Model file for the job. Use its own axes, mm. A direction names the side the tool comes from. Round coordinates to 2 decimals unless told otherwise and drop trailing zeros. Write each loop counter-clockwise with the first axis right and the second up, starting at its lowest first coordinate (ties: lowest second). Pieces come first, ordered by that corner, then holes. Notation, with made-up numbers: (-17.5, 22) - (8.5, 22) arc R25 ccw to (8.5, 38) - close; hole circle Ø1 at (17.25, -33). An arc over 180 degrees is marked (long way). Answer as a JSON object with one key per item and string values. Group by question number.
Autodesk Fusion 360 part; units mm, degrees
sketch "Sketch1" plane through (0, 0, 0) normal (0, 1, 0) x (1, 0, 0)
  line L0 (0, 0) -> (203.5, 0)
  line L1 (209.5, -6) -> (209.5, -39)
  line L2 (204.5, -14) -> (204.5, -36)
  line L3 (204.5, -40) -> (208.5, -40)
  line L4 (204.5, -40) -> (198, -40)
  line L5 (203.5, -37) -> (201, -37)
  line L6 (200, -36) -> (200, -35.5)
  line L7 (199, -34.5) -> (198, -34.5)
  line L8 (197, -35.5) -> (197, -39)
  arc A0 (200, -35.5) -> (199, -34.5) centre (199, -35.5) ccw
  arc A1 (198, -34.5) -> (197, -35.5) centre (198, -35.5) ccw
  arc A2 (200, -36) -> (201, -37) centre (201, -36) ccw
  arc A3 (203.5, -37) -> (204.5, -36) centre (203.5, -36) ccw
  arc A4 (197, -39) -> (198, -40) centre (198, -39) ccw
  arc A5 (208.5, -40) -> (209.5, -39) centre (208.5, -39) ccw
  line L9 (0, -8) -> (198.5, -8)
  arc A6 (204.5, -14) -> (198.5, -8) centre (198.5, -14) ccw
  arc A7 (209.5, -6) -> (203.5, 0) centre (203.5, -6) ccw
  line L10 (185, 0) -> (185, -8)
  point P0 (204.5, 0)
  point P1 (209.5, 0)
  point P2 (209.5, -40)
  point P3 (200, -37)
  point P4 (200, -34.5)
  point P5 (197, -34.5)
  point P6 (197, -40)
  dimension "d14" = 5
  dimension "d15" = 40
  dimension "d16" = 7.5
  dimension "d17" = 5.5
  dimension "d18" = 3
  dimension "d20" = 2.5
  dimension "d21" = 1
  dimension "d22" = 1
  dimension "d23" = 1
  dimension "d24" = 1
  dimension "d26" = 6
  dimension "d27" = 6
extrude "Extrude1" add sketch "Sketch1" along normal blind 29
(1) Drill centre lines: line 1 (Z direction, x = 198.5, y = 11); line 2 (Z direction, x = 196.25, y = 15.25); line 3 (X direction, y = 12.75, z = 14.5). Where is each one in solid material? Low to high. Write a range as from..to.
(2) Slice it at B-B (y = 8.25). Write the cut outline in (x, z), then the cut area to 3 significant figures.
(3) Slice it at A-A (z = 35). Write the cut outline in (x, y), then the cut area to 3 significant figures.
(4) 3-axis set-ups, long thin cutter, end or side, ignore diameter. For faces 1 (the cylindrical face through (204.215, 14.297, 36.699)), 2 (the flat face through (197, 14, 37)), 3 (the flat face through (198.5, 14.3, 34.5)): which of +Z, -Z, +X, -X, +Y, -Y reach the whole face in a straight line?
(5) Slice it at C-C (x = 188). Write the cut outline in (y, z), then the cut area to 3 significant figures.
(6) Slice it at D-D (z = 16). Write the cut outline in (x, y).
(7) Pull direction X, two halves, no side cores. Call faces 4 (the cylindrical face through (197.285, 14.297, 34.801)), 5 (the cylindrical face through (199.699, 14.297, 34.785)), 6 (the cylindrical face through (209.215, 14.297, 39.699)): pulls with the +X half, pulls with the -X half, needs draft (parallel to the pull), parting line crosses it, or undercut.
(8) Flat gauge pins, fed straight in: pin 1 (4 mm diameter, centred on y = 11, z = 37, fed in from -X); pin 2 (4 mm diameter, centred on x = 190.5, y = 7.5, fed in from +Z); pin 3 (5 mm diameter, centred on x = 201, y = 13.5, fed in from -Z); pin 4 (4 mm diameter, centred on y = 11.5, z = 29, fed in from -X). Where does each tip first touch, or does it go through?
Answer:
{
 "1": {"line 1": "0..8, 34.5..40", "line 2": "0..8", "line 3": "204.5..209.5"},
 "2": {"outline": "(185, 0) - (203.5, 0) arc R6 ccw to (209.5, 6) - (209.5, 39) arc R1 ccw to (208.5, 40) - (198, 40) arc R1 ccw to (197, 39) - (197, 35.5) arc R1 ccw to (198, 34.5) - (199, 34.5) arc R1 ccw to (200, 35.5) - (200, 36) arc R1 cw to (201, 37) - (203.5, 37) arc R1 cw to (204.5, 36) - (204.5, 14) arc R6 cw to (198.5, 8) - (185, 8) - close", "area": "386 mm²"},
 "3": {"outline": "(197.13, 0) - (199.87, 0) - (199.87, 29) - (197.13, 29) - close; (204.5, 0) - (209.5, 0) - (209.5, 29) - (204.5, 29) - close", "area": "224 mm²"},
 "4": {"face 1": "+Y, -Y", "face 2": "+Z, -X, +Y, -Y", "face 3": "-X, +Y, -Y"},
 "5": {"outline": "(0, 0) - (29, 0) - (29, 8) - (0, 8) - close", "area": "232 mm²"},
 "6": {"outline": "(204.5, 0) - (209.5, 0) - (209.5, 29) - (204.5, 29) - close"},
 "7": {"face 4": "pulls with the -X half", "face 5": "undercut", "face 6": "pulls with the +X half"},
 "8": {"pin 1": "x = 197", "pin 2": "z = 8", "pin 3": "z = 0", "pin 4": "x = 204.5"}
}
